For this review, take the finished solid that the model builds, in its own axes (mm). Coordinates: 2 decimals unless noted, no trailing zeros. Loops run counter-clockwise (first coordinate to the right, second up) from the corner with the lowest first, then second, coordinate; pieces in that order, holes last. Notation, with made-up numbers: (-4.5, 22.25) - (43.5, 22.25) arc R19 cw to (43.5, 47.25) - close; hole circle Ø6 at (65, -31). An arc over 180 degrees is marked (long way). Use one line per item in the form item = value. Start each with the question number.
1. Add section B-B on z = 18. Give the boundary of the cut face in (x, y), and give its area (3 significant figures).
2. To check wall thickness, follow probe 1 along Z at (x, y) = (0, -28.25); probe 2 along X at (y, z) = (-30, 0); probe 3 along Z at (x, y) = (0, -29). State the ranges of each line that lie inside material, in increasing order.
3. Add section A-A on y = -29.5. Give the boundary of the cut face in (x, z), and give its area (3 significant figures).
4. Add section C-C on x = 10. Give the boundary of the cut face in (y, z), and give its area (3 significant figures).
5. For pin 1 Ø12 at (x, z) = (-21, 6.5) entering from -Y; pin 2 Ø6 at (x, z) = (22, 4.5) entering from -Y; pin 3 Ø4 at (x, z) = (-7.5, -17) entering from -Y, all flat-tipped, find the tip position at first contact; note any pin that passes through.
6. Add section D-D on y = -22.5. Give the boundary of the cut face in (x, z).
```python
from build123d import *

# Parameters (mm, degrees)
SKETCH2_R           = 33.8
CUT_EXTRUDE1_DEPTH  = 19.1
SKETCH20_R          = 0.5
CUT_EXTRUDE13_DEPTH = 43.087409044


with BuildPart() as part:
    # Sketch1 → Revolve1 (revolve)
    with BuildSketch(Plane.XY, mode=Mode.PRIVATE) as revolve1_sk:
        with BuildLine():
            Line((0, -33.8), (0, 0))
            Line((0, 0), (33.8, 0))
            ThreePointArc((33.8, 0), (23.900209204, -23.900209204), (0, -33.8))
        make_face()
    revolve(revolve1_sk.sketch.rotate(Axis((0, -33.8, 0), (0, 1, 0)), 180), axis=Axis((0, -33.8, 0), (0, 1, 0)))

    # Sketch2 → Cut-Extrude1 (cut)
    with BuildSketch(Plane(origin=(0, 0, 0), x_dir=(1, 0, 0), z_dir=(0, 1, 0))):
        Circle(SKETCH2_R)
    extrude(amount=-CUT_EXTRUDE1_DEPTH, mode=Mode.SUBTRACT)

    # Sketch20 → Cut-Extrude13 (cut, through all)
    with BuildSketch(Plane(origin=(0, -19.1, 0), x_dir=(1, 0, 0), z_dir=(0, 1, 0))):
        with Locations(Location((0, 0, 0), (0, 0, 270))):
            Circle(SKETCH20_R)
    extrude(amount=-CUT_EXTRUDE13_DEPTH, mode=Mode.SUBTRACT)


solid = part.part
```
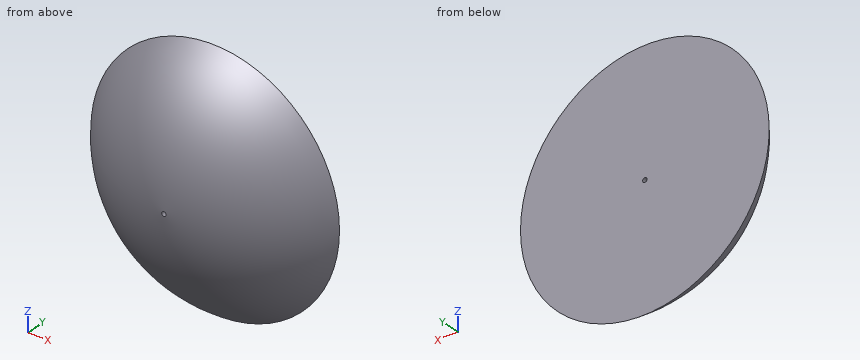
Conclusion:
q1.outline = (-21.3, -19.1) arc R28.61 ccw to (21.3, -19.1) - close
q1.area = 280 mm^2
q2.probe_1 = -18.56 to -0.5, 0.5 to 18.56
q2.probe_2 = -15.57 to -0.5, 0.5 to 15.57
q2.probe_3 = -17.36 to -0.5, 0.5 to 17.36
q3.outline = circle Ø33 at (0, 0); hole circle Ø1 at (0, 0)
q3.area = 854 mm^2
q4.outline = (-19.1, -26.03) - (-19.1, 26.03) arc R32.29 ccw to start
q4.area = 480 mm^2
q5.pin_1 = -29.78
q5.pin_2 = -27.64
q5.pin_3 = -29.45
q6.outline = circle Ø50.45 at (0, 0); hole circle Ø1 at (0, 0)
